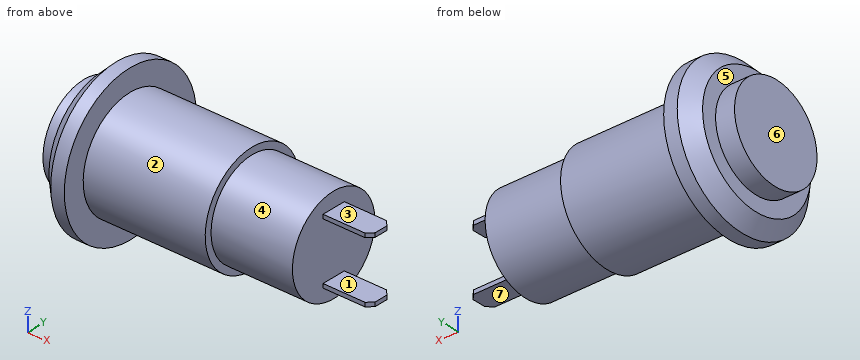
```python
from build123d import *

# Parameters (mm, degrees)
CHAMFER_1_SIZE  = 1
SKETCH_4_W      = 0.3
SKETCH_4_H      = 1.8
EXTRUDE_1_DEPTH = 3.5
CHAMFER_2_SIZE  = 0.4


with BuildPart() as part:
    # 草图2 → 旋转2 (revolve)
    with BuildSketch(Plane.XY, mode=Mode.PRIVATE) as revolve_2_sk:
        Polygon((0, 0), (0, -3.5), (1.4, -3.5), (1.4, -5.60259245), (3.4, -5.60259245), (3.4, -4), (12.4, -4), (12.4, -3.5), (18.4, -3.5), (18.4, 0), align=None)
    revolve(revolve_2_sk.sketch.rotate(Axis((-3.092696523, 0, 0), (1, 0, 0)), 270), axis=Axis((-3.092696523, 0, 0), (1, 0, 0)))

    # 倒角1
    chamfer_1_edges = [part.edges().sort_by_distance(p)[0] for p in [
        (1.4, 0, -5.60259245),
    ]]
    chamfer(chamfer_1_edges, length=CHAMFER_1_SIZE)

    # 草图4 → 凸台-拉伸1 (add)
    with BuildSketch(Plane(origin=(18.4, 0, 0), x_dir=(0, 0, -1), z_dir=(1, 0, 0))):
        with Locations((-2.25, 0)):
            Rectangle(SKETCH_4_W, SKETCH_4_H)
        with Locations((2.25, 0)):
            Rectangle(SKETCH_4_W, SKETCH_4_H)
    extrude(amount=EXTRUDE_1_DEPTH)

    # 倒角2
    chamfer_2_edges = [part.edges().sort_by_distance(p)[0] for p in [
        (21.9, -0.9, 2.25),
        (21.9, 0.9, 2.25),
        (21.9, -0.9, -2.25),
        (21.9, 0.9, -2.25),
    ]]
    chamfer(chamfer_2_edges, length=CHAMFER_2_SIZE)


solid = part.part
```
Input: part model. Units: mm. Frame: model coordinates. Face numbers are marked on the shaded views. A direction names the side the tool comes from. Give positions to 0.01 mm unless a question says otherwise; leave off trailing zeros. Order: outer loops, then holes, each group sorted by start corner. A loop starts at its lowest first (then second) coordinate and runs counter-clockwise, first axis right, second up. Notation, with made-up numbers: (48.25, -24.75) - (54.25, -24.75) arc R22 ccw to (54.25, -17.75) - close; hole circle Ø2 at (-21.5, 19). An arc over 180 degrees is marked (long way). One line per item, written item: value.
1. Reachability of the marked faces 4, 5, 6 and 7 from +Z, -Z, +X, -X, +Y, -Y: full face, straight path, thin tool, end or side. Return the list, or none.
Determined:
face 4: +X
face 5: -X
face 6: +Z, -Z, -X, +Y, -Y
face 7: -Z, +X, +Y, -Y
2. Cut plane C-C, the plane x = 5.75. Output: boundary loops of the cut face in (y, z), and give its area (3 significant figures).
Determined:
outline: circle Ø8 at (0, 0)
area: 50.3 mm2
3. Line query: probe 1 along Z at (x, y) = (20.75, -0.25); probe 2 along X at (y, z) = (-1, 0.75); probe 3 along X at (y, z) = (-1.75, 4.25). Output: solid intervals per line, ascending.
Determined:
probe 1: -2.4 to -2.1, 2.1 to 2.4
probe 2: 0 to 18.4
probe 3: 1.4 to 3.4
4. Cut plane B-B, the plane z = 0. Output: boundary loops of the cut face in (x, y).
Determined:
outline: (0, -3.5) - (1.4, -3.5) - (1.4, -4.6) - (2.4, -5.6) - (3.4, -5.6) - (3.4, -4) - (12.4, -4) - (12.4, -3.5) - (18.4, -3.5) - (18.4, 3.5) - (12.4, 3.5) - (12.4, 4) - (3.4, 4) - (3.4, 5.6) - (2.4, 5.6) - (1.4, 4.6) - (1.4, 3.5) - (0, 3.5) - close
5. Draft query along Z for the marked faces 1, 2 and 3. Return one class per face: released by +Z, released by -Z, zero draft, split by the parting line, or undercut.
Determined:
face 1: undercut
face 2: split by the parting line
face 3: released by +Z
6. Cut plane A-A, the plane y = 0. Output: boundary loops of the cut face in (x, z).
Determined:
outline: (0, -3.5) - (1.4, -3.5) - (1.4, -4.6) - (2.4, -5.6) - (3.4, -5.6) - (3.4, -4) - (12.4, -4) - (12.4, -3.5) - (18.4, -3.5) - (18.4, -2.4) - (21.9, -2.4) - (21.9, -2.1) - (18.4, -2.1) - (18.4, 2.1) - (21.9, 2.1) - (21.9, 2.4) - (18.4, 2.4) - (18.4, 3.5) - (12.4, 3.5) - (12.4, 4) - (3.4, 4) - (3.4, 5.6) - (2.4, 5.6) - (1.4, 4.6) - (1.4, 3.5) - (0, 3.5) - close
7. Pin query (flat end, axial travel): pin 1 Ø0.5 at (x, y) = (19.5, 0) entering from +Z; pin 2 Ø1 at (x, y) = (6, -3) entering from -Z; pin 3 Ø4 at (x, z) = (17.5, 4) entering from +Y. Return the tip coordinate at first contact, or that it passes through.
Determined:
pin 1: z = 2.4
pin 2: z = -3.12
pin 3: y = 2.87
